Model file for the job. Use its own axes, mm. A direction names the side the tool comes from. Round coordinates to 2 decimals unless told otherwise and drop trailing zeros. Loops run counter-clockwise (first coordinate to the right, second up) from the corner with the lowest first, then second, coordinate; pieces in that order, holes last. Notation, with made-up numbers: (67.25, 2.5) - (104.25, 2.5) arc R14 ccw to (104.25, 27.5) - close; hole circle Ø3 at (76.5, 33). An arc over 180 degrees is marked (long way). Use one line per item in the form item = value.
from build123d import *

# Parameters (mm, degrees)
SKETCH1_R           = 12.5
BOSS_EXTRUDE1_DEPTH = 85
SKETCH2_R           = 3.95
BOSS_EXTRUDE2_DEPTH = 35
BOSS_EXTRUDE3_START = 35
SKETCH3_R           = 3.95
BOSS_EXTRUDE3_DEPTH = 35


with BuildPart() as part:
    # Sketch1 → Boss-Extrude1 (new body)
    with BuildSketch(Plane.XY):
        Circle(SKETCH1_R)
    extrude(amount=-BOSS_EXTRUDE1_DEPTH)

    # Sketch2 → Boss-Extrude2 (add)
    with BuildSketch(Plane.XY):
        Circle(SKETCH2_R)
    extrude(amount=BOSS_EXTRUDE2_DEPTH)

    # Sketch3 → Boss-Extrude3 (add)
    with BuildSketch(Plane(origin=(0, 0, -85), x_dir=(-1, 0, 0), z_dir=(0, 0, -1)).offset(BOSS_EXTRUDE3_START)):
        with Locations(Location((0, 0, 0), (0, 0, 180))):
            Circle(SKETCH3_R)
    extrude(amount=-BOSS_EXTRUDE3_DEPTH)


solid = part.part
1. Tool access for faces 1 (the flat face through (-3, 3, 0)), 2 (the cylindrical face through (11.923, 3.755, -41.905)), 3 (the flat face through (-3, 3, -85)): list every direction of +Z, -Z, +X, -X, +Y, -Y with a clear straight run to the whole face (end or side of a thin tool).
Geometry check:
face_1 = +Z
face_2 = +Z, -Z
face_3 = -Z
2. Wall check: probe 1 along Z at (x, y) = (0.25, -4.75); probe 2 along Y at (x, z) = (0.75, -79.5); probe 3 along X at (y, z) = (1.25, -91). Give the ranges that are in metal, low to high.
Geometry check:
probe_1 = -85 to 0
probe_2 = -12.48 to 12.48
probe_3 = -3.75 to 3.75
3. Flat gauge pins, fed straight in: pin 1 (4 mm diameter, centred on x = 7.5, y = 0, fed in from +Z); pin 2 (8 mm diameter, centred on x = -4.5, z = -75, fed in from -Y); pin 3 (3 mm diameter, centred on x = -5.5, y = 3, fed in from -Z); pin 4 (7.5 mm diameter, centred on x = -4, y = 2, fed in from -Z). Where does each tip first touch, or does it go through?
Geometry check:
pin_1 = 0
pin_2 = -12.49
pin_3 = -85
pin_4 = -120
4. Cut at D-D, the plane x = 7.5. Give the cut face in (y, z).
Geometry check:
outline = (-10, -85) - (10, -85) - (10, 0) - (-10, 0) - close
5. Cut at A-A, the plane y = 0. Give the cut face in (x, z).
Geometry check:
outline = (-12.5, -85) - (-3.95, -85) - (-3.95, -120) - (3.95, -120) - (3.95, -85) - (12.5, -85) - (12.5, 0) - (3.95, 0) - (3.95, 35) - (-3.95, 35) - (-3.95, 0) - (-12.5, 0) - close
6. Cut at C-C, the plane z = -15.5. Give the cut face in (x, y).
Geometry check:
outline = circle Ø25 at (0, 0)
